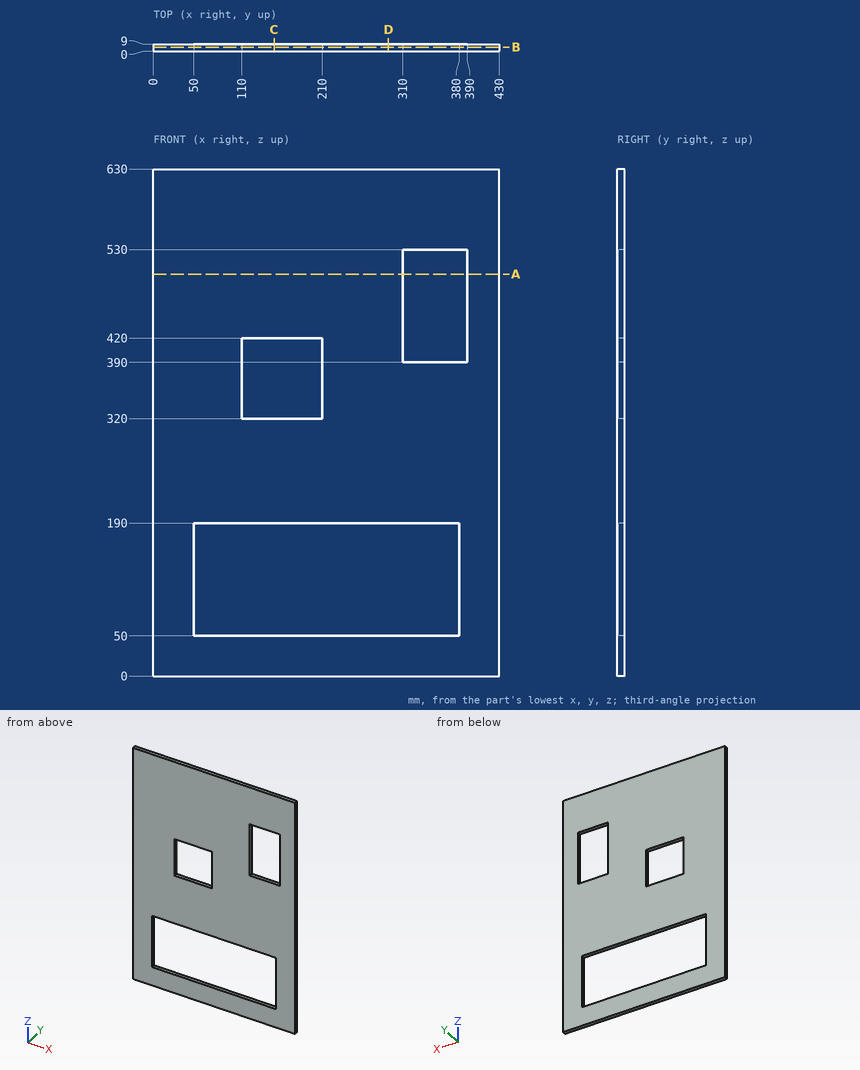
Geometry: see drawing. Coordinates: mm, zero at the bounding-box minimum. Round coordinates to 2 decimals unless told otherwise and drop trailing zeros. Write each loop counter-clockwise with the first axis right and the second up, starting at its lowest first coordinate (ties: lowest second). Pieces come first, ordered by that corner, then holes. Notation, with made-up numbers: M -10.5,38.25 L 34.5,38.25 A18 cw 34.5,73.25 Z; hole C -37,-18.75 d6. An arc over 180 degrees is marked long. Answer as a JSON object with one key per item and string values. Group by question number.
(1) Section query D-D on x = 292. Output: boundary loops of the cut face in (y, z), then the cut area to 3 significant figures.
(2) Section query C-C on x = 150. Output: boundary loops of the cut face in (y, z).
(3) Section query B-B on y = 5.25. Output: boundary loops of the cut face in (x, z), then the cut area to 4 significant figures.
(4) Section query A-A on z = 499.5. Output: boundary loops of the cut face in (x, y).
(5) Ray query, line 1 (Z direction, x = 131.5, y = 6); line 2 (X direction, y = 3, z = 412); line 3 (Z direction, x = 346.5, y = 2.25). Return the intervals inside material, ascending. Write a range as [from, to].
Computed values:
{
 "1": {"outline": "M 0,0 L 9,0 L 9,50 L 0,50 Z; M 0,190 L 9,190 L 9,630 L 0,630 Z", "area": "4,410 mm^2"},
 "2": {"outline": "M 0,0 L 9,0 L 9,50 L 0,50 Z; M 0,190 L 9,190 L 9,320 L 0,320 Z; M 0,420 L 9,420 L 9,630 L 0,630 Z"},
 "3": {"outline": "M 0,0 L 430,0 L 430,630 L 0,630 Z; hole M 50,50 L 380,50 L 380,190 L 50,190 Z; hole M 110,320 L 210,320 L 210,420 L 110,420 Z; hole M 310,390 L 390,390 L 390,530 L 310,530 Z", "area": "203,500 mm^2"},
 "4": {"outline": "M 0,0 L 310,0 L 310,9 L 0,9 Z; M 390,0 L 430,0 L 430,9 L 390,9 Z"},
 "5": {"line 1": "[0, 50], [190, 320], [420, 630]", "line 2": "[0, 110], [210, 310], [390, 430]", "line 3": "[0, 50], [190, 390], [530, 630]"}
}
